from build123d import *

# Parameters (mm, degrees)
SKETCH1_R            = 3
CRANK_BODY_DEPTH     = 4.5
PIN_SHAFT_BODY_DEPTH = 3
SKETCH4_R            = 2.3
PIN_SHAFT_DEPTH      = 7
SKETCH1_2_OUTSIDE_W  = 11.382
SKETCH1_2_OUTSIDE_H  = 14.382
SKETCH1_2_OUTSIDE_R  = 3
SMOOTHING_CUTS_DEPTH = 5
SKETCH5_R            = 4
CUT_EXTRUDE1_DEPTH   = 7


with BuildPart() as part:
    # Sketch1 → crank_body (new body)
    with BuildSketch(Plane(origin=(0, 0, 0), x_dir=(1, 0, 0), z_dir=(0, 1, 0))):
        Circle(SKETCH1_R)
    extrude(amount=CRANK_BODY_DEPTH)

    # Sketch3 → pin_shaft_body (add, symmetric)
    with BuildSketch(Plane(origin=(0, 0, 0), x_dir=(0, 0, -1), z_dir=(1, 0, 0))):
        with BuildLine():
            Line((-3, 5), (-3, 4.5))
            Line((-3, 4.5), (3, 4.5))
            Line((3, 4.5), (3, 5))
            Line((3, 5), (2.828427125, 5))
            ThreePointArc((2.828427125, 5), (0, 13), (-2.828427125, 5))
            Line((-2.828427125, 5), (-3, 5))
        make_face()
    pin_shaft_body = extrude(amount=PIN_SHAFT_BODY_DEPTH, both=True)

    # Sketch4 → pin_shaft (cut, through all)
    with BuildSketch(Plane(origin=(3, 0, 0), x_dir=(0, 0, -1), z_dir=(1, 0, 0))):
        with Locations((0, 8.5)):
            Circle(SKETCH4_R)
    extrude(amount=-PIN_SHAFT_DEPTH, mode=Mode.SUBTRACT)

    # Sketch1<2> outside → smoothing_cuts (cut)
    with BuildSketch(Plane(origin=(0, 0, 0), x_dir=(1, 0, 0), z_dir=(0, 1, 0))):
        Rectangle(SKETCH1_2_OUTSIDE_W, SKETCH1_2_OUTSIDE_H)
        Circle(SKETCH1_2_OUTSIDE_R, mode=Mode.SUBTRACT)
    smoothing_cuts = extrude(amount=SMOOTHING_CUTS_DEPTH, mode=Mode.SUBTRACT)

    # Mirror1: pin_shaft_body, smoothing_cuts across plane
    add(pin_shaft_body.mirror(Plane(origin=(0, 2.5, 0), x_dir=(0, 0, 1), z_dir=(0, -1, 0))))
    add(smoothing_cuts.mirror(Plane(origin=(0, 2.5, 0), x_dir=(0, 0, 1), z_dir=(0, -1, 0))), mode=Mode.SUBTRACT)

    # Sketch5 → Cut-Extrude1 (cut, through all)
    with BuildSketch(Plane(origin=(3, 0, 0), x_dir=(0, 0, -1), z_dir=(1, 0, 0))):
        with Locations((0, -3.5)):
            Circle(SKETCH5_R)
    extrude(amount=-CUT_EXTRUDE1_DEPTH, mode=Mode.SUBTRACT)


solid = part.part
The listing builds one solid part. Answer for the finished solid, in the listing's coordinates (mm). A direction names the side the tool comes from. Give positions to 0.01 mm unless a question says otherwise; leave off trailing zeros. Loops run counter-clockwise (first coordinate to the right, second up) from the corner with the lowest first, then second, coordinate; pieces in that order, holes last. Notation, with made-up numbers: M 29,82 L 33,82 A24 ccw 33,117 Z; hole C -34.75,32 d9. An arc over 180 degrees is marked long. Answer as CSV lines item,"result".
Item 1: The part is cut by section B-B (x = -2.5). Give the vertices of the cut face in (y, z), and give its area (3 significant figures).
Values follow:
outline,"M 0,-2.83 L 0,-1.94 A4 cw long 0,1.94 L 0,2.83 A4.5 ccw long Z; M 0.14,-1.66 L 5,-1.66 L 5,-2.83 A4.5 ccw long 5,2.83 L 5,1.66 L 0.14,1.66 A4 cw Z; hole C 8.5,0 d4.6"
area,"69.2 mm^2"
Item 2: Which of the six approach directions +Z, -Z, +X, -X, +Y, -Y give full straight-line access (tool end or side, diameter ignored) to faces 4 (the flat face through (2.4, 0, 2.5)), 5 (the flat face through (-2.4, 5, 2.2)), 6 (the flat face through (-2.5, 5, -2.2))?
Values follow:
face 4,"+Z, +X"
face 5,"+Z, -X"
face 6,"-Z, -X"
Item 3: The part is cut by section A-A (y = -3.5). Give the vertices of the cut face in (x, z).
Values follow:
outline,"M -3,-4.5 L 3,-4.5 L 3,-4 L -3,-4 Z; M -3,4 L 3,4 L 3,4.5 L -3,4.5 Z"
Item 4: Given pin 1 Ø1.6 at (x, z) = (2, 2) entering from -Y; pin 2 Ø1 at (x, z) = (2.5, 2.5) entering from +Y; pin 3 Ø0.6 at (x, z) = (-2.5, 1) entering from -Y, each flat-ended and moving along its own axis, determine where each tip first touches the part or whether it passes through.
Values follow:
pin 1,"stops at y = -7.84"
pin 2,"stops at y = 12.53"
pin 3,"stops at y = -7.95"
Item 5: The part is cut by section C-C (z = -2.5). Give the vertices of the cut face in (x, y).
Values follow:
outline,"M -3,-7.24 L 3,-7.24 L 3,-6.62 L -3,-6.62 Z; M -3,-0.38 L 3,-0.38 L 3,0 L 1.66,0 L 1.66,5 L 3,5 L 3,12.24 L -3,12.24 L -3,5 L -1.66,5 L -1.66,0 L -3,0 Z"
Item 6: Straight lines are drawn through the part: line 1 along Y through (x, z) = (-1, 0); line 2 along Y through (x, z) = (0.75, -1); line 3 along Z through (x, y) = (2.75, -7). For each, find the intervals that lie inside material, in ascending order. Write a range as [from, to].
Values follow:
line 1,"y = [-8, -7.5], [0.5, 6.2], [10.8, 13]"
line 2,"y = [-7.89, -7.37], [0.37, 6.43], [10.57, 12.89]"
line 3,"z = [-2.83, -1.94], [1.94, 2.83]"
Item 7: The part is cut by section D-D (x = 1.25). Give the vertices of the cut face in (y, z), and give its area (3 significant figures).
Values follow:
outline,"M 0,-2.83 L 0,-2.73 L 5,-2.73 L 5,-2.83 A4.5 ccw long 5,2.83 L 5,2.73 L 0,2.73 L 0,2.83 A4.5 ccw long Z; hole C -3.5,0 d8; hole C 8.5,0 d4.6"
area,"79.9 mm^2"
Item 8: The mould has two halves that part along Z. Classify faces 1 (the flat face through (2.4, 0, -2.5)), 2 (the cylindrical face through (0, -8, 0)), 3 (the cylindrical face through (0.042, -7.405, 0.867)): released by +Z, released by -Z, zero draft, split by the parting line, or undercut.
Values follow:
face 1,"zero draft"
face 2,"split by the parting line"
face 3,"undercut"
